Here's how the part is built. I have some questions about the finished solid (model axes, mm). A direction names the side the tool comes from. Round coordinates to 2 decimals unless told otherwise and drop trailing zeros. Write each loop counter-clockwise with the first axis right and the second up, starting at its lowest first coordinate (ties: lowest second). Pieces come first, ordered by that corner, then holes. Notation, with made-up numbers: (24, -9.5) -> (77, -9.5) arc R14 cw to (77, 5.5) -> close; hole circle Ø5 at (28.25, 6.5). An arc over 180 degrees is marked (long way). Put each result on its own line as item: value. Start each with the question number.
1. I need wall thicknesses on probe 1 along X at (y, z) = (1.45, -5); probe 2 along Y at (x, z) = (-23.5, 2); probe 3 along X at (y, z) = (16.75, -6.75). Which ranges of each line are inside material? Lowest first, please. Write a range as from..to.
2. Which directions (+Z, -Z, +X, -X, +Y, -Y) give clear straight access to the entire face, cutting with the end or side of a thin tool? Please do faces 5 (the face through (29, 4, -5)), 6 (the face through (0, 26, 0)), 7 (the face through (21, 1, 0)).
3. Suppose I cut it at D-D (y = 24.75). Please give me the cut outline in (x, z), then the cut area to 3 significant figures.
4. Suppose I cut it at B-B (z = 0). Please give me the cut outline in (x, y).
5. Suppose I cut it at A-A (y = 17.75). Please give me the cut outline in (x, z).
6. For pin 1 (3 mm diameter, centred on x = 17.5, z = -2.5, fed in from -Y), with a flat end and sliding along its axis, tell me the tip position at first contact or that it passes through.
7. Suppose I cut it at C-C (x = 9.3). Please give me the cut outline in (y, z), then the cut area to 3 significant figures.
8. We'd pull the mould along Y, two halves only. Please class faces 1 (the face through (-26, 2, -6)), 2 (the face through (29, 4, 5)), 3 (the face through (-26, 0, 0)), 4 (the face through (-23.12, 0.99, -3.71)): +Y half, -Y half, draft (parallel to the pull), parting line (faces both ways), or undercut.
```python
from build123d import *

# Parameters (mm, degrees)
RESSALTO_EXTRUS_O1_DEPTH = 9
ESBO_O2_R                = 1.75
CORTE_EXTRUS_O1_DEPTH    = 16
RESSALTO_EXTRUS_O3_DEPTH = 1.5
ESBO_O6_R                = 1.6
CORTE_EXTRUS_O2_DEPTH    = 3
ESBO_O7_W                = 5
ESBO_O7_H                = 10
CORTE_EXTRUS_O3_DEPTH    = 10
RESSALTO_EXTRUS_O4_START = 3.2
ESBO_O8_W                = 8
ESBO_O8_H                = 18
ESBO_O8_R                = 1.75
RESSALTO_EXTRUS_O4_DEPTH = 3


with BuildPart() as part:
    # Esboço1 → Ressalto-extrusão1 (new, symmetric)
    with BuildSketch(Plane.XY):
        Polygon((-21, 0), (-31, 0), (-31, 29), (31, 29), (31, 0), (21, 0), (21, 2), (29, 2), (29, 26), (-29, 26), (-29, 2), (-21, 2), align=None)
    extrude(amount=RESSALTO_EXTRUS_O1_DEPTH, both=True)

    # Esboço2 → Corte-extrusão1 (cut)
    with BuildSketch(Plane.XZ):
        with Locations(Location((-24.3, -5, 0), (0, 0, 270))):
            Circle(ESBO_O2_R)
        with Locations(Location((-24.3, 5, 0), (0, 0, 270))):
            Circle(ESBO_O2_R)
        with Locations(Location((24.3, 5, 0), (0, 0, 270))):
            Circle(ESBO_O2_R)
        with Locations(Location((24.3, -5, 0), (0, 0, 270))):
            Circle(ESBO_O2_R)
    extrude(amount=-CORTE_EXTRUS_O1_DEPTH, mode=Mode.SUBTRACT)

    # Esboço4 → Ressalto-extrusão3 (add, symmetric)
    with BuildSketch(Plane.XY):
        Polygon((-21, 2), (-29, 10), (-29, 2), align=None)
        Polygon((21, 2), (29, 2), (29, 10), align=None)
    extrude(amount=RESSALTO_EXTRUS_O3_DEPTH, both=True)

    # Esboço6 → Corte-extrusão2 (cut)
    with BuildSketch(Plane(origin=(0, 29, 0), x_dir=(1, 0, 0), z_dir=(0, 1, 0))):
        with Locations(Location((9.3, 0, 0), (0, 0, 270))):
            Circle(ESBO_O6_R)
    extrude(amount=-CORTE_EXTRUS_O2_DEPTH, mode=Mode.SUBTRACT)

    # Esboço7 → Corte-extrusão3 (cut)
    with BuildSketch(Plane(origin=(31, 0, 0), x_dir=(0, 0, -1), z_dir=(1, 0, 0))):
        with Locations((0, 19)):
            Rectangle(ESBO_O7_W, ESBO_O7_H)
    extrude(amount=-CORTE_EXTRUS_O3_DEPTH, mode=Mode.SUBTRACT)

    # Esboço8 → Ressalto-extrusão4 (add)
    # profile 1 of 2: a face of its own
    with BuildSketch(Plane(origin=(0, 2, 0), x_dir=(1, 0, 0), z_dir=(0, 1, 0)).offset(RESSALTO_EXTRUS_O4_START)):
        with Locations((-25, 0)):
            Rectangle(ESBO_O8_W, ESBO_O8_H)
        with Locations(Location((-24.3, -5, 0), (0, 0, 90))):
            Circle(ESBO_O8_R, mode=Mode.SUBTRACT)
        with Locations(Location((-24.3, 5, 0), (0, 0, 90))):
            Circle(ESBO_O8_R, mode=Mode.SUBTRACT)
    # profile 2 of 2: a face of its own
    with BuildSketch(Plane(origin=(0, 2, 0), x_dir=(1, 0, 0), z_dir=(0, 1, 0)).offset(RESSALTO_EXTRUS_O4_START)):
        with Locations((25, 0)):
            Rectangle(ESBO_O8_W, ESBO_O8_H)
        with Locations(Location((24.3, -5, 0), (0, 0, 90))):
            Circle(ESBO_O8_R, mode=Mode.SUBTRACT)
        with Locations(Location((24.3, 5, 0), (0, 0, 90))):
            Circle(ESBO_O8_R, mode=Mode.SUBTRACT)
    extrude(amount=RESSALTO_EXTRUS_O4_DEPTH)


solid = part.part
```
Verdict:
1. probe 1: x = -31..-26.05, -22.55..-21, 21..22.55, 26.05..31
1. probe 2: y = 0..2, 5.2..8.2, 26..29
1. probe 3: x = -31..-29, 29..31
2. face 5: -Z
2. face 6: +Z, -Z
2. face 7: +Z, -Z, -Y
3. outline: (-31, -9) -> (-29, -9) -> (-29, 9) -> (-31, 9) -> close; (29, -9) -> (31, -9) -> (31, 9) -> (29, 9) -> close
3. area: 72.0 mm^2
4. outline: (-31, 0) -> (-21, 0) -> (-21, 2) -> (-24.2, 5.2) -> (-21, 5.2) -> (-21, 8.2) -> (-27.2, 8.2) -> (-29, 10) -> (-29, 26) -> (7.7, 26) -> (7.7, 29) -> (-31, 29) -> close; (10.9, 26) -> (29, 26) -> (29, 24) -> (31, 24) -> (31, 29) -> (10.9, 29) -> close; (21, 0) -> (31, 0) -> (31, 14) -> (29, 14) -> (29, 10) -> (27.2, 8.2) -> (21, 8.2) -> (21, 5.2) -> (24.2, 5.2) -> (21, 2) -> close
5. outline: (-31, -9) -> (-29, -9) -> (-29, 9) -> (-31, 9) -> close; (29, -9) -> (31, -9) -> (31, -2.5) -> (29, -2.5) -> close; (29, 2.5) -> (31, 2.5) -> (31, 9) -> (29, 9) -> close
6. pin 1: stops at y = 26
7. outline: (26, -9) -> (29, -9) -> (29, -1.6) -> (26, -1.6) -> close; (26, 1.6) -> (29, 1.6) -> (29, 9) -> (26, 9) -> close
7. area: 44.4 mm^2
8. face 1: undercut
8. face 2: undercut
8. face 3: -Y half
8. face 4: draft
